The listing builds one solid part. Answer for the finished solid, in the listing's coordinates (mm). Face numbers are marked on the shaded views. Give positions to 0.01 mm unless a question says otherwise; leave off trailing zeros. Loops run counter-clockwise (first coordinate to the right, second up) from the corner with the lowest first, then second, coordinate; pieces in that order, holes last.
Item 1: Section D-D, the plane x = -19 is taken. Give the vertices of the cut face in (y, z), and give its area (3 significant figures).
Item 2: Section C-C, the plane y = -1.25 is taken. Give the vertices of the cut face in (x, z), and give its area (3 significant figures).
Item 3: Each of these flat-tipped pins is pushed along its axis until it touches: pin 1 Ø0.6 at (y, z) = (-3.5, -3) entering from -X; pin 2 Ø2.5 at (x, y) = (20, -3.5) entering from +Z; pin 3 Ø2 at (y, z) = (-0.5, -15) entering from +X. Where does it stop, or does it pass through?
Item 4: Consider line 1 along Z through (x, y) = (0, -2.2); line 2 along Z through (x, y) = (22, -2.25); line 3 along X through (y, z) = (-0.8, 0). Determine where each line is inside the solid, lowest interval first.
Item 5: Section A-A, the plane z = 0 is taken. Give the vertices of the cut face in (x, y), and give its area (3 significant figures).
Item 6: Section B-B, the plane x = -1 is taken. Give the vertices of the cut face in (y, z).
Item 7: The mould has two halves that part along Z. Classify the marked faces 1, 2 and 3: pulls with the +Z half, pulls with the -Z half, needs draft (parallel to the pull), parting line crosses it, or undercut.
from build123d import *
from build123d.topology import SkipClean

# Parameters (mm, degrees)
SKETCH1_R                 = 1.25
SKETCH1_R_2               = 2.45
BOSS_EXTRUDE1_DEPTH       = 2
BOSS_EXTRUDE2_START       = -3
BOSS_EXTRUDE2_OUTLINE_R   = 4.9
BOSS_EXTRUDE2_OUTLINE_R_2 = 2.45
BOSS_EXTRUDE2_DEPTH       = 1
SKETCH1_5_W               = 13.43962311
SKETCH1_5_H               = 2
BOSS_EXTRUDE3_DEPTH       = 7
FILLET1_R                 = 10
FILLET2_R                 = 5
FILLET3_R                 = 1.2
FILLET4_R                 = 1.2


# Read off the part's stored shape, not the designer's step: Boss-Extrude2
with BuildPart() as part:
    # Sketch1 → Boss-Extrude1 (new body)
    with BuildSketch(Plane(origin=(0, 0, 0), x_dir=(1, 0, 0), z_dir=(0, 1, 0))):
        with BuildLine():
            ThreePointArc((1.939071943, 4.5), (0.989949494, 4.79895822), (0, 4.9))
            Line((0, 4.9), (0, 26.132651094))
            ThreePointArc((0, 26.132651094), (-16.812473395, -20.006403764), (25.742289199, 4.5))
            Line((25.742289199, 4.5), (1.939071943, 4.5))
        make_face()
        with Locations(Location((14.206057781, -5.961892897, 0), (0, 0, 270))):
            Circle(SKETCH1_R, mode=Mode.SUBTRACT)
        with Locations(Location((21.786269316, -5.961892897, 0), (0, 0, 270))):
            Circle(SKETCH1_R, mode=Mode.SUBTRACT)
        with Locations(Location((0, 0, 0), (0, 0, 270))):
            Circle(SKETCH1_R_2, mode=Mode.SUBTRACT)
    extrude(amount=-BOSS_EXTRUDE1_DEPTH)

    # Boss-Extrude2 outline → Boss-Extrude2 (add)
    with SkipClean():  # the faces are left unmerged after this step: merging them gives an invalid solid
        with BuildSketch(Plane(origin=(0, 0, 0), x_dir=(1, 0, 0), z_dir=(0, 1, 0)).offset(BOSS_EXTRUDE2_START)):
            Circle(BOSS_EXTRUDE2_OUTLINE_R)
            Circle(BOSS_EXTRUDE2_OUTLINE_R_2, mode=Mode.SUBTRACT)
        extrude(amount=BOSS_EXTRUDE2_DEPTH)
    add(part.part.scale(1), mode=Mode.REPLACE)  # the faces are merged on a copy

    # Sketch1<5> → Boss-Extrude3 (add)
    with BuildSketch(Plane(origin=(0, 0, 0), x_dir=(1, 0, 0), z_dir=(0, 1, 0))):
        with Locations((18.609497145, 3.5)):
            Rectangle(SKETCH1_5_W, SKETCH1_5_H)
        with Locations((18.609497145, -3.5)):
            Rectangle(SKETCH1_5_W, SKETCH1_5_H)
    extrude(amount=-BOSS_EXTRUDE3_DEPTH)

    # Fillet1
    # the kernel refuses this fillet: 10 mm, written as the material it adds along each edge
    with BuildSketch(Plane(origin=(0, 0, -4.9), x_dir=(0, 0, -1), z_dir=(0, -1, 0))) as fillet1_piece_1:
        with BuildLine():
            CenterArc((6.145813687, 10), FILLET1_R, 222.155184251, 47.844815749)
            ThreePointArc((-1.26748409, 3.288590604), (-0.32783815, 1.762196362), (0, 0))
            Line((0, 0), (6.145813687, 0))
        make_face()
    extrude(amount=2)

    # Fillet2
    fillet2_edges = [part.edges().sort_by_distance(p)[0] for p in [
        (0, -1, -26.132651094),
    ]]
    fillet(fillet2_edges, radius=FILLET2_R)

    # Fillet3
    fillet3_edges = [part.edges().sort_by_distance(p)[0] for p in [
        (18.609497145, -7, 4.5),
    ]]
    fillet(fillet3_edges, radius=FILLET3_R)

    # Fillet4
    fillet4_edges = [part.edges().sort_by_distance(p)[0] for p in [
        (18.609497145, -7, -4.5),
    ]]
    fillet(fillet4_edges, radius=FILLET4_R)


solid = part.part
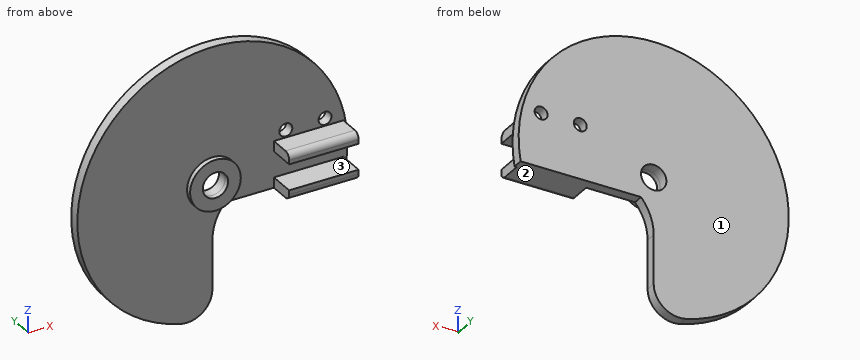
Worked answers:
1. outline: (-2, -17.94) - (0, -17.94) - (0, 17.94) - (-2, 17.94) - close
1. area: 71.8 mm2
2. outline: (-6.18, -25.39) arc R5 ccw to (0, -20.53) - (0, -11.05) arc R10 cw to (2.44, -4.5) - (25.74, -4.5) arc R26.13 ccw (long way) to start; hole circle Ø4.9 at (0, 0); hole circle Ø2.5 at (14.21, 5.96); hole circle Ø2.5 at (21.79, 5.96)
2. area: 1,690 mm2
3. pin 1: stops at x = 11.89
3. pin 2: stops at z = 4.5
3. pin 3: stops at x = 0
4. line 1: z = -4.9 to -2.45, 2.45 to 4.9
4. line 2: z = -4.5 to -2.5, 2.5 to 4.5
4. line 3: x = -26.13 to -2.45, 2.45 to 26.13
5. outline: (-26.13, -2) - (-4.9, -2) - (-4.9, -3) - (-2.45, -3) - (-2.45, 0) - (-26.13, 0) - close; (2.45, -3) - (4.9, -3) - (4.9, -2) - (26.13, -2) - (26.13, 0) - (2.45, 0) - close
5. area: 99.6 mm2
6. outline: (-3, -4.8) - (-2, -4.8) - (-2, -23.53) - (0, -23.53) - (0, -2.24) - (-3, -2.24) - close; (-3, 2.24) - (0, 2.24) - (0, 26.11) - (-2, 26.11) - (-2, 4.8) - (-3, 4.8) - close
7. face 1: needs draft
7. face 2: pulls with the -Z half
7. face 3: undercut
